Geometry check sheet. Reference: drawing and pictorial views, mm from the part's lowest x, y, z. A direction names the side the tool comes from. Give positions to 0.01 mm unless a question says otherwise; leave off trailing zeros. Loops run counter-clockwise (first coordinate to the right, second up) from the corner with the lowest first, then second, coordinate; pieces in that order, holes last. Notation, with made-up numbers: (37, -30.5) -> (49, -30.5) arc R24 ccw to (49, -19.5) -> close; hole circle Ø11 at (27.25, 55.5). An arc over 180 degrees is marked (long way). Write item = value, one per line. Start each with the question number.
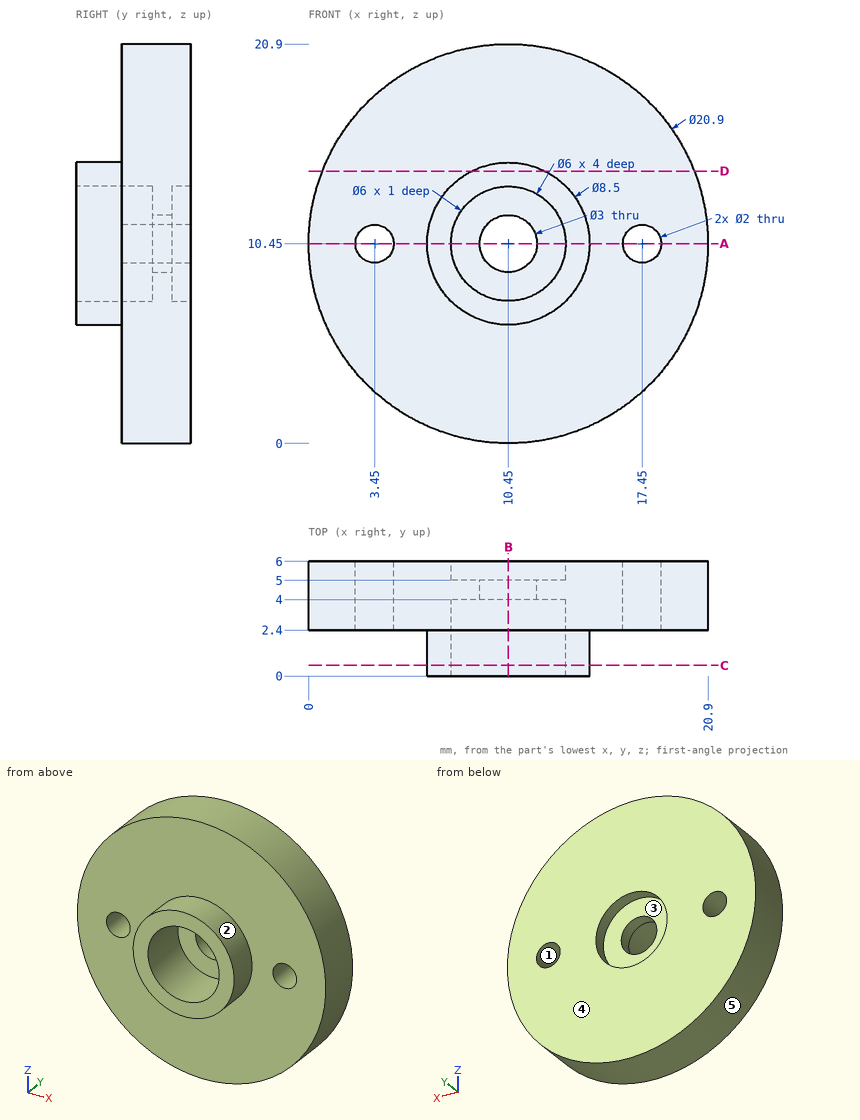
1) Tool access check on the marked faces 1 and 2. Record the directions out of +Z, -Z, +X, -X, +Y, -Y that give a thin tool (end or side, any length) a straight path to the whole face; none if there is none.
2) Thickness scan on line 1 (X direction, y = 4.55, z = 10.45); line 2 (X direction, y = 5.2, z = 10.45); line 3 (Y direction, x = 6.5, z = 12.75). Record the ranges inside material, lowest first.
3) Section check A-A (z = 10.45). Enter the section's corners in (x, y).
4) Draft check along X on the marked faces 3, 4 and 5. Enter one of: released by +X, released by -X, zero draft, split by the parting line, or undercut.
5) Section check C-C (y = 0.55). Enter the section's corners in (x, z), plus the area to 3 significant figures.
6) Section check D-D (z = 14.25). Enter the section's corners in (x, y), plus the area to 3 significant figures.
7) Depth check by flat-ended pin: pin 1 Ø2 at (y, z) = (2.5, 15) entering from -X; pin 2 Ø3 at (x, z) = (9.5, 9.5) entering from +Y; pin 3 Ø3 at (x, z) = (15.5, 2.5) entering from -Y; pin 4 Ø2.5 at (x, z) = (3.45, 10.45) entering from +Y. Enter the tip coordinate at first touch or a pass-through.
8) Section check B-B (x = 10.45). Enter the section's corners in (y, z).
Check result:
q1.face_1 = +Y, -Y
q1.face_2 = -Y
q2.line_1 = 0 to 2.45, 4.45 to 8.95, 11.95 to 16.45, 18.45 to 20.9
q2.line_2 = 0 to 2.45, 4.45 to 7.45, 13.45 to 16.45, 18.45 to 20.9
q2.line_3 = 2.4 to 6
q3.outline = (0, 2.4) -> (2.45, 2.4) -> (2.45, 6) -> (0, 6) -> close; (4.45, 2.4) -> (6.2, 2.4) -> (6.2, 0) -> (7.45, 0) -> (7.45, 4) -> (8.95, 4) -> (8.95, 5) -> (7.45, 5) -> (7.45, 6) -> (4.45, 6) -> close; (11.95, 4) -> (13.45, 4) -> (13.45, 0) -> (14.7, 0) -> (14.7, 2.4) -> (16.45, 2.4) -> (16.45, 6) -> (13.45, 6) -> (13.45, 5) -> (11.95, 5) -> close; (18.45, 2.4) -> (20.9, 2.4) -> (20.9, 6) -> (18.45, 6) -> close
q4.face_3 = undercut
q4.face_4 = zero draft
q4.face_5 = split by the parting line
q5.outline = circle Ø8.5 at (10.45, 10.45); hole circle Ø6 at (10.45, 10.45)
q5.area = 28.5 mm2
q6.outline = (0.72, 2.4) -> (8.55, 2.4) -> (8.55, 0) -> (12.35, 0) -> (12.35, 2.4) -> (20.18, 2.4) -> (20.18, 6) -> (0.72, 6) -> close
q6.area = 79.2 mm2
q7.pin_1 = 0.62
q7.pin_2 = 5
q7.pin_3 = 2.4
q7.pin_4 = 6
q8.outline = (0, 6.2) -> (2.4, 6.2) -> (2.4, 0) -> (6, 0) -> (6, 7.45) -> (5, 7.45) -> (5, 8.95) -> (4, 8.95) -> (4, 7.45) -> (0, 7.45) -> close; (0, 13.45) -> (4, 13.45) -> (4, 11.95) -> (5, 11.95) -> (5, 13.45) -> (6, 13.45) -> (6, 20.9) -> (2.4, 20.9) -> (2.4, 14.7) -> (0, 14.7) -> close
